Work out the finished part from the listing and answer in its coordinate system (mm). Coordinates: 2 decimals unless noted, no trailing zeros. Order: outer loops, then holes, each group sorted by start corner. A loop starts at its lowest first (then second) coordinate and runs counter-clockwise, first axis right, second up. Notation, with made-up numbers: (54.5, -27) - (95.5, -27) arc R31 ccw to (95.5, -1) - close; hole circle Ø2 at (0.25, 63). An arc over 180 degrees is marked (long way). Use CSV: the item, a comma, the result in double quotes. Start each with the question number.
from build123d import *

# Parameters (mm, degrees)
SKIZZE2_R = 3.114282512


with BuildPart() as part:
    # Austragung1: sweep along a path in Skizze1
    with BuildLine(Plane(origin=(0, 0, 0), x_dir=(1, 0, 0), z_dir=(0, 1, 0))) as austragung1_path:
        ThreePointArc((0, -82.442660512), (-33.108990695, -75.502231804), (-60.643425983, -55.849504539))
        ThreePointArc((-60.643425983, -55.849504539), (-64.562830296, -49.572910331), (-65.931764421, -42.300814045))
        Line((-65.931764421, -42.300814045), (-65.931764421, 42.300814045))
        ThreePointArc((-65.931764421, 42.300814045), (-64.562830296, 49.572910331), (-60.643425983, 55.849504539))
        ThreePointArc((-60.643425983, 55.849504539), (-33.108990695, 75.502231804), (0, 82.442660512))
    # Skizze2 → Austragung1 (sweep)
    with BuildSketch(Plane(origin=(0, 0, 0), x_dir=(0, 0, -1), z_dir=(1, 0, 0))):
        with Locations((-82.442660512, 0)):
            Circle(SKIZZE2_R)
    sweep(path=austragung1_path.line)

    # Spiegeln1: part across plane


with BuildPart() as part_1:
    add(part.part)
    add(part.part.mirror(Plane(origin=(0, 0, 82.442660512), x_dir=(0, 0, 1), z_dir=(1, 0, 0))))


solid = part_1.part
1) Straight lines are drawn through the part: line 1 (X direction, y = 0.5, z = -6); line 2 (X direction, y = 0, z = 17.5); line 3 (Z direction, x = 12, y = 0.75). For each, find the intervals that lie inside material, in ascending order. Write a range as [from, to].
2) Flat-ended cylindrical pins translate along their axes: P1, Ø3, axis at x = -7.5, y = 0, coming from the -Z side; P2, Ø3, axis at y = 0.5, z = -19.5, coming from the -X side; P3, Ø1, axis at x = 18.5, y = 0.5, coming from the +Z side. Find the tip coordinate at first contact, or state that the pin passes through.
3) The part is cut by section B-B on y = -2. Determine the outline of the cut face in (x, z), plus the area to 3 significant figures.
4) The part is cut by section A-A on z = -14. Determine the outline of the cut face in (x, y), plus the area to 3 significant figures.
Answer key:
1,line 1,"[-69.01, -62.86], [62.86, 69.01]"
1,line 2,"[-69.05, -62.82], [62.82, 69.05]"
1,line 3,"[-84.62, -78.51], [78.51, 84.62]"
2,P1,"z = -85.35"
2,P2,"x = -69.05"
2,P3,"z = 83.62"
3,outline,"(-68.32, -42.3) arc R22.39 ccw to (-62.4, -57.47) arc R84.83 ccw to (62.4, -57.47) arc R22.39 ccw to (68.32, -42.3) - (68.32, 42.3) arc R22.39 ccw to (62.4, 57.47) arc R84.83 ccw to (-62.4, 57.47) arc R22.39 ccw to (-68.32, 42.3) - close; hole (-63.54, -42.3) arc R17.61 ccw to (-58.89, -54.23) arc R80.06 ccw to (58.89, -54.23) arc R17.61 ccw to (63.54, -42.3) - (63.54, 42.3) arc R17.61 ccw to (58.89, 54.23) arc R80.06 ccw to (-58.89, 54.23) arc R17.61 ccw to (-63.54, 42.3) - close"
3,area,"2,390 mm^2"
4,outline,"circle Ø6.23 at (-65.93, 0); circle Ø6.23 at (65.93, 0)"
4,area,"60.9 mm^2"
